Here's how the part is built. I have some questions about the finished solid (model axes, mm). Face numbers are marked on the shaded views. A direction names the side the tool comes from. Coordinates: 2 decimals unless noted, no trailing zeros. Loops run counter-clockwise (first coordinate to the right, second up) from the corner with the lowest first, then second, coordinate; pieces in that order, holes last. Notation, with made-up numbers: M 8,0.25 L 67,0.25 A13 ccw 67,4.25 Z; hole C 58.25,-29.75 d11. An arc over 180 degrees is marked long. Use CSV: the item, a comma, the result in double quotes. Start each with the question number.
Q1. If we section it at B-B (x = 32): Please give me the cut outline in (y, z).
Q2. Which directions (+Z, -Z, +X, -X, +Y, -Y) give clear straight access to the entire face, cutting with the end or side of a thin tool? Please do the marked faces 4 and 5.
Q3. If we section it at D-D (x = 0): Please give me the cut outline in (y, z).
Q4. If we section it at A-A (z = 6): Please give me the cut outline in (x, y).
Q5. Please list where these lines run through material, in increasing order: probe 1 along Y at (x, z) = (-0.5, 23.5); probe 2 along Z at (x, y) = (-27, 36.5); probe 3 along Y at (x, z) = (-3, 27). Write a range as [from, to].
Q6. If we section it at C-C (y = 0): Please give me the cut outline in (x, z), and give its area (3 significant figures).
Q7. If we mould it in two halves opening along Y, with no side actions, what happens to the marked faces 1, 2 and 3? For each: +Y half, -Y half, draft (parallel to the pull), parting line (faces both ways), or undercut.
Q8. For pin 1 Ø8 at (x, y) = (19.5, 2.5) entering from -Z; pin 2 Ø0.7 at (y, z) = (5.5, 21.5) entering from -X; pin 3 Ø1 at (x, y) = (23.5, -15.5) entering from +Z; pin 4 Ø6 at (x, z) = (11.5, 10.5) entering from -Y, each with a flat end and sliding along its axis, tell me the tip position at first contact or that it passes through.
from build123d import *

# Parameters (mm, degrees)
F0_R           = 50
F1_DEPTH       = 2
F3_R           = 10
F4_DEPTH       = 1.5
F5_D           = 6.4
F5_CSINK_D     = 13.44
F5_CSINK_ANGLE = 90
F6_W           = 18
F6_H           = 1.45
F7_DEPTH       = 30
F9_DEPTH       = 25
F10_T1_DEPTH   = 39.192646775


# Not quite as in the source:
# - a fillet or chamfer that OpenCascade refuses, or shapes differently, is made with other operations: its cross-section is extruded or revolved along the edge and cut away or added


with BuildPart() as f1:
    # F0 (on Top) → F1 (new body)
    with BuildSketch(Plane.XY):
        Circle(F0_R)
    extrude(amount=F1_DEPTH)

    # F3 (on face) → F4 (join)
    with BuildSketch(Plane(origin=(0, 0, 0), x_dir=(1, 0, 0), z_dir=(0, 0, -1))):
        with Locations((31.9376476109, 0)):
            Circle(F3_R)
        with Locations((-32.1291722357, 0)):
            Circle(F3_R)
    extrude(amount=F4_DEPTH)

    # F5 (through all)
    with Locations(Plane.XY.offset(2)):
        with Locations((-32, 0), (32, 0)):
            CounterSinkHole(F5_D / 2, F5_CSINK_D / 2, counter_sink_angle=F5_CSINK_ANGLE)

    # F6 (on face) → F7 (join)
    with BuildSketch(Plane.XY.offset(2)):
        with Locations((0, 5.725)):
            Rectangle(F6_W, F6_H)
        with Locations((0, -5.725)):
            Rectangle(F6_W, F6_H)
    extrude(amount=F7_DEPTH)

    # F8 (on face) → F9 (cut)
    with BuildSketch(Plane.XZ.offset(6.45)):
        Polygon((9, 32), (-9, 32), (9, 28), align=None)
    extrude(amount=-F9_DEPTH, mode=Mode.SUBTRACT)

    # F10: chamfer of 4 x 1.4558809371 on 2 edges, made by hand

    # F10_s2 → F10_t1 (cut)
    with BuildSketch(Plane(origin=(-25.4826184945, 0, 5.6628041099), x_dir=(0, 1, 0), z_dir=(0.9761870602, 0, -0.2169304578))):
        Polygon((6.45, 25.2856118055), (4.9941190629, 29.2856118055), (6.45, 29.2856118055), align=None)
        Polygon((-6.45, 25.2856118055), (-4.9941190629, 29.2856118055), (-6.45, 29.2856118055), align=None)
    extrude(amount=F10_T1_DEPTH, mode=Mode.SUBTRACT)


solid = f1.part
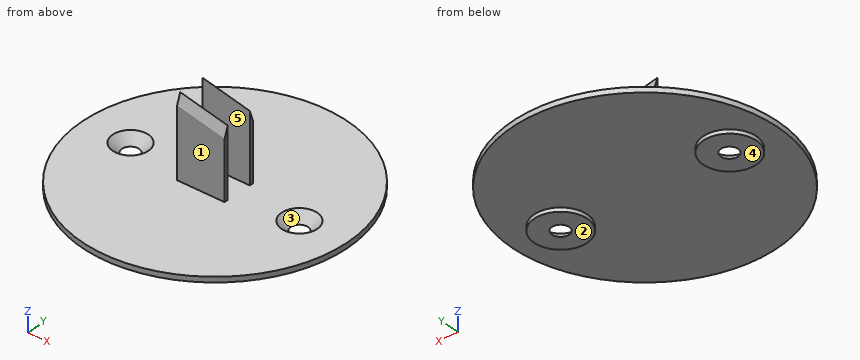
Results below:
1,outline,"M -38.42,0 L -10,0 L -10,-1.5 L -3.22,-1.5 L -6.72,2 L -38.42,2 Z; M 3.22,-1.5 L 10,-1.5 L 10,0 L 38.42,0 L 38.42,2 L 6.72,2 Z"
2,face 4,"-Z, +X, -X, +Y, -Y"
2,face 5,"+Z, +X, -X"
3,outline,"M -50,0 L 50,0 L 50,2 L 6.45,2 L 6.45,25.9 L 5,29.98 L 5,2 L -5,2 L -5,29.98 L -6.45,25.9 L -6.45,2 L -50,2 Z"
4,outline,"M -9,-6.45 L 9,-6.45 L 9,-5 L -9,-5 Z; M -9,5 L 9,5 L 9,6.45 L -9,6.45 Z"
5,probe 1,"[-6.45, -5], [5, 6.45]"
5,probe 2,"[0, 2]"
5,probe 3,"[-6.3, -5], [5, 6.3]"
6,outline,"M -50,0 L -42.13,0 L -42.13,-1.5 L -35.22,-1.5 L -38.72,2 L -50,2 Z; M -28.78,-1.5 L -22.13,-1.5 L -22.13,0 L 21.94,0 L 21.94,-1.5 L 28.78,-1.5 L 25.28,2 L -25.28,2 Z; M 35.22,-1.5 L 41.94,-1.5 L 41.94,0 L 50,0 L 50,2 L 38.72,2 Z"
6,area,"190 mm^2"
7,face 1,"-Y half"
7,face 2,"draft"
7,face 3,"undercut"
8,pin 1,"z = -1.5"
8,pin 2,"x = -9"
8,pin 3,"z = 2"
8,pin 4,"y = -6.45"
